```python
from build123d import *

# Parameters (mm, degrees)
SKETCH1_W           = 28.194
SKETCH1_H           = 2.54
BOSS_EXTRUDE1_DEPTH = 6.477
SKETCH2_W           = 28.194
SKETCH2_H           = 16.256
SKETCH2_W_2         = 23.114
SKETCH2_H_2         = 11.176
BOSS_EXTRUDE2_DEPTH = 1.27
SKETCH3_W           = 21.59
SKETCH3_H           = 2.54
SKETCH3_W_2         = 2.54
SKETCH3_H_2         = 18.796
SKETCH3_W_3         = 13.97
CUT_EXTRUDE1_DEPTH  = 3.302
SKETCH4_R           = 2.54
BOSS_EXTRUDE3_DEPTH = 3.302
FILLET4_R           = 1.27


with BuildPart() as part:
    # Sketch1 → Boss-Extrude1 (new body)
    with BuildSketch(Plane.XY):
        with Locations((-4.067663462, 13.041923077)):
            Rectangle(SKETCH1_W, SKETCH1_H)
        Polygon((-18.164663462, 14.311923077), (-20.704663462, 14.311923077), (-20.704663462, -7.024076923), (12.569336538, -7.024076923), (12.569336538, 14.311923077), (10.029336538, 14.311923077), (10.029336538, 11.771923077), (10.029336538, -4.484076923), (-18.164663462, -4.484076923), (-18.164663462, 11.771923077), align=None)
    extrude(amount=BOSS_EXTRUDE1_DEPTH)

    # Sketch2 → Boss-Extrude2 (add)
    with BuildSketch(Plane(origin=(0, 0, 0), x_dir=(-1, 0, 0), z_dir=(0, 0, -1))):
        with Locations((4.067663462, 3.643923077)):
            Rectangle(SKETCH2_W, SKETCH2_H)
        with Locations((4.067663462, 3.643923077)):
            Rectangle(SKETCH2_W_2, SKETCH2_H_2, mode=Mode.SUBTRACT)
    extrude(amount=-BOSS_EXTRUDE2_DEPTH)

    # Sketch3 → Cut-Extrude1 (cut)
    with BuildSketch(Plane.XY.offset(6.477)):
        with Locations((-9.909663462, 13.041923077)):
            Rectangle(SKETCH3_W, SKETCH3_H)
        with Locations((11.299336538, 4.913923077)):
            Rectangle(SKETCH3_W_2, SKETCH3_H_2)
        with Locations((11.299336538, -5.754076923)):
            Rectangle(SKETCH3_W_2, SKETCH3_H)
        with Locations((3.044336538, -5.754076923)):
            Rectangle(SKETCH3_W_3, SKETCH3_H)
    extrude(amount=-CUT_EXTRUDE1_DEPTH, mode=Mode.SUBTRACT)

    # Sketch4 → Boss-Extrude3 (add)
    with BuildSketch(Plane(origin=(0, 14.311923077, 0), x_dir=(1, 0, 0), z_dir=(0, 1, 0))):
        with BuildLine():
            Line((-14.227663462, 10.16), (-14.227663462, 0))
            Line((-14.227663462, 0), (6.092336538, 0))
            Line((6.092336538, 0), (6.092336538, 10.16))
            ThreePointArc((6.092336538, 10.16), (-4.067663462, 20.32), (-14.227663462, 10.16))
        make_face()
        with Locations(Location((-4.067663462, 10.16, 0), (0, 0, 270))):
            Circle(SKETCH4_R, mode=Mode.SUBTRACT)
    extrude(amount=-BOSS_EXTRUDE3_DEPTH)

    # Fillet4
    fillet4_edges = [part.edges().sort_by_distance(p)[0] for p in [
        (-4.067663462, 11.009923077, 0),
        (6.092336538, 12.660923077, 0),
        (-14.227663462, 12.660923077, 0),
        (-15.624663462, 9.231923077, 0.635),
        (-15.624663462, -1.944076923, 0.635),
        (7.489336538, -1.944076923, 0.635),
        (7.489336538, 9.231923077, 0.635),
    ]]
    fillet(fillet4_edges, radius=FILLET4_R)


solid = part.part
```
Build history of the part. All positions in model axes, mm. A direction names the side the tool comes from. Round coordinates to 2 decimals unless told otherwise and drop trailing zeros. Loops run counter-clockwise (first coordinate to the right, second up) from the corner with the lowest first, then second, coordinate; pieces in that order, holes last. Notation, with made-up numbers: M 18.5,24 L 53.5,24 A14 cw 53.5,30 Z; hole C -17.5,31.25 d5. An arc over 180 degrees is marked long. Answer as CSV lines item,"result".
1. Cut at B-B on y = -3.5. Write the cut outline in (x, z) (3 decimals).
Resolved:
outline,"M -20.705,0 L 12.569,0 L 12.569,3.175 L 10.029,3.175 L 10.029,1.27 L -18.165,1.27 L -18.165,6.477 L -20.705,6.477 Z"
2. Wall check: probe 1 along Y at (x, z) = (-13.5, 1.5); probe 2 along X at (y, z) = (13.2, -10.16); probe 3 along Y at (x, z) = (1, 0.25). Give the ranges that are in metal, low to high. Write a range as [from, to].
Resolved:
probe 1,"y = [-7.02, -4.48], [11.77, 14.31]"
probe 2,"x = [-14.23, -6.61], [-1.53, 6.09]"
probe 3,"y = [-7.02, -1.94], [9.23, 14.31]"
3. Cut at C-C on z = -9.25. Write the cut outline in (x, y), then the cut area to 3 significant figures.
Resolved:
outline,"M -14.23,11.01 L -6.44,11.01 L -6.44,14.31 L -14.23,14.31 Z; M -1.7,11.01 L 6.09,11.01 L 6.09,14.31 L -1.7,14.31 Z"
area,"51.4 mm²"
4. Cut at A-A on y = 2.25. Write the cut outline in (x, z) (3 decimals).
Resolved:
outline,"M -20.705,0 L -15.625,0 L -15.625,1.27 L -18.165,1.27 L -18.165,6.477 L -20.705,6.477 Z; M 7.489,0 L 12.569,0 L 12.569,3.175 L 10.029,3.175 L 10.029,1.27 L 7.489,1.27 Z"
5. 3-axis set-ups, long thin cutter, end or side, ignore diameter. For faces 4 (the flat face through (-19, 11.772, 5)), 5 (the cylindrical face through (7.127, 8.85, 0.644)), 6 (the flat face through (10.4, -0.3, 3.175)): which of +Z, -Z, +X, -X, +Y, -Y reach the whole face in a straight line?
Resolved:
face 4,"+Z, -X, +Y"
face 5,"+Z, -Z"
face 6,"+Z, +X, -Y"
6. Flat gauge pins, fed straight in: P1, Ø3, axis at y = -6, z = 5, coming from the +X side; P2, Ø3, axis at x = -19.5, z = 5.5, coming from the +Y side; P3, Ø6.5, axis at x = -9.5, y = 3, coming from the -Z side; P4, Ø5.5, axis at x = -7, z = -12, coming from the -Y side. Where does each tip first touch, or does it go through?
Resolved:
P1,"stops at x = -3.94"
P2,"stops at y = 11.77"
P3,"passes through"
P4,"stops at y = 11.01"
7. Cut at D-D on x = -9. Write the cut outline in (y, z) (3 decimals), then the cut area to 3 significant figures.
Resolved:
outline,"M -7.024,0 L -1.944,0 L -1.944,1.27 L -4.484,1.27 L -4.484,6.477 L -7.024,6.477 Z; M 9.232,0 L 9.74,0 A1.27 cw 11.01,-1.27 L 11.01,-19.042 L 14.312,-19.042 L 14.312,3.175 L 11.772,3.175 L 11.772,1.27 L 9.232,1.27 Z"
area,"94.2 mm²"
8. Two-plate mould, pull along X, no slides. Class faces 1 (the flat face through (-4, 14.312, -7)), 2 (the flat face through (10.029, 13, 5)), 3 (the flat face through (-4, -1.944, 1)): released by +X, released by -X, zero draft, split by the parting line, or undercut.
Resolved:
face 1,"zero draft"
face 2,"released by +X"
face 3,"undercut"
